from build123d import *

# Parameters (mm, degrees)
F0_R     = 30
F1_DEPTH = 14
F2_T     = -2.5
F3_R     = 3
F4_DEPTH = 2.5
F5_SIZE  = 2


with BuildPart() as f1:
    # F0 (on Front) → F1 (new body)
    with BuildSketch(Plane.XZ):
        Circle(F0_R)
    extrude(amount=F1_DEPTH)

    # F2
    f2_openings = [f1.faces().sort_by_distance(p)[0] for p in [
        (0, 0, 0),
    ]]
    offset(amount=F2_T, openings=f2_openings)

    # F3 (on face) → F4 (cut, through all)
    with BuildSketch(Plane.XZ.offset(14)):
        with Locations((0, -24)):
            Circle(F3_R)
        with Locations((-24, 0)):
            Circle(F3_R)
        with Locations((24, 0)):
            Circle(F3_R)
        with Locations((0, 24)):
            Circle(F3_R)
    extrude(amount=-F4_DEPTH, mode=Mode.SUBTRACT)

    # F5
    f5_edges = [f1.edges().sort_by_distance(p)[0] for p in [
        (-30, -14, 0),
    ]]
    chamfer(f5_edges, length=F5_SIZE)


solid = f1.part
The listing builds one solid part. Answer for the finished solid, in the listing's coordinates (mm). A direction names the side the tool comes from. Give positions to 0.01 mm unless a question says otherwise; leave off trailing zeros. Write each loop counter-clockwise with the first axis right and the second up, starting at its lowest first coordinate (ties: lowest second). Pieces come first, ordered by that corner, then holes. Notation, with made-up numbers: (-39.75, 61) -> (14.25, 61) arc R16 ccw to (14.25, 82) -> close; hole circle Ø5 at (28, 27). An arc over 180 degrees is marked (long way). Use a Markdown table: item, result.
(1) Determine the mould class of faces 1 (the cylindrical face through (-29.97, -5.92, 1.32)), 2 (the flat face through (0, -11.5, 0)), 3 (the cylindrical face through (-27, -13, 0)), 4 (the flat face through (0, -14, 0)) for opening direction Z: released by +Z, released by -Z, zero draft, split by the parting line, or undercut.
Return value:
| item | result |
|---|---|
| face 1 | split by the parting line |
| face 2 | undercut |
| face 3 | undercut |
| face 4 | zero draft |
(2) Flat-ended cylindrical pins translate along their axes: P1, Ø2, axis at y = -10, z = -22.5, coming from the -X side; P2, Ø5.5, axis at x = -24, z = 0, coming from the +Y side; P3, Ø1.5, axis at y = -12.5, z = -23.5, coming from the +X side; P4, Ø5, axis at x = -2, z = -15.5, coming from the +Y side. Find the tip coordinate at first contact, or state that the pin passes through.
Return value:
| item | result |
|---|---|
| P1 | x = -20.92 |
| P2 | through |
| P3 | x = 19.33 |
| P4 | y = -11.5 |
(3) For faces 5 (the cylindrical face through (-5.961, -5.67, -26.846)), 6 (the cylindrical face through (-0.65, -12.77, 21.07)), determine the directions among +Z, -Z, +X, -X, +Y, -Y from which every point of the face is accessible in a straight line to the end or side of a thin tool.
Return value:
| item | result |
|---|---|
| face 5 | +Y |
| face 6 | +Y, -Y |
(4) Section A-A, the plane z = 0 is taken. Determine the outline of the cut face in (x, y), then the cut area to 4 significant figures.
Return value:
| item | result |
|---|---|
| outline | (-30, -12) -> (-28, -14) -> (-27, -14) -> (-27, -11.5) -> (-27.5, -11.5) -> (-27.5, 0) -> (-30, 0) -> close; (-21, -14) -> (21, -14) -> (21, -11.5) -> (-21, -11.5) -> close; (27, -14) -> (28, -14) -> (30, -12) -> (30, 0) -> (27.5, 0) -> (27.5, -11.5) -> (27, -11.5) -> close |
| area | 173.5 mm2 |
(5) Section B-B, the plane x = 0 is taken. Determine the outline of the cut face in (y, z).
Return value:
| item | result |
|---|---|
| outline | (-14, -28) -> (-12, -30) -> (0, -30) -> (0, -27.5) -> (-11.5, -27.5) -> (-11.5, -27) -> (-14, -27) -> close; (-14, -21) -> (-11.5, -21) -> (-11.5, 21) -> (-14, 21) -> close; (-14, 27) -> (-11.5, 27) -> (-11.5, 27.5) -> (0, 27.5) -> (0, 30) -> (-12, 30) -> (-14, 28) -> close |
(6) Section C-C, the plane y = -4.75 is taken. Determine the outline of the cut face in (x, z), then the cut area to 3 significant figures.
Return value:
| item | result |
|---|---|
| outline | circle Ø60 at (0, 0); hole circle Ø55 at (0, 0) |
| area | 452 mm2 |
(7) Find the intervals of material crossed by probe 1 along Z at (x, y) = (0, -12.5); probe 2 along Y at (x, z) = (7, -20.5); probe 3 along Z at (x, y) = (-0.5, -5), in increasing order. Write a range as from..to.
Return value:
| item | result |
|---|---|
| probe 1 | -29.5..-27, -21..21, 27..29.5 |
| probe 2 | -14..-11.5 |
| probe 3 | -30..-27.5, 27.5..30 |
